```python
from build123d import *

# Parameters (mm, degrees)
SKETCH1_R           = 1.5
SKETCH1_R_2         = 1
BOSS_EXTRUDE1_DEPTH = 5
FILLET1_R           = 20
CUT_EXTRUDE1_START  = -2.5
CUT_EXTRUDE1_DEPTH  = 2.5
FILLET5_R           = 15
FILLET6_R           = 4
CHAMFER1_SIZE       = 1.5


with BuildPart() as part:
    # Sketch1 → Boss-Extrude1 (new body)
    with BuildSketch(Plane(origin=(0, 0, 0), x_dir=(1, 0, 0), z_dir=(0, 1, 0))):
        with BuildLine():
            Line((0.6, -5.969924623), (50.1, -0.994987437))
            Line((50.1, -0.994987437), (60.292075574, -4.699254638))
            ThreePointArc((60.292075574, -4.699254638), (66.917086627, -0.906785038), (62.080644677, 4.999349601))
            Line((62.080644677, 4.999349601), (0.105263158, 5.999076568))
            ThreePointArc((0.105263158, 5.999076568), (-2.95430253, 5.222269292), (-5.196152423, 3))
            Line((-5.196152423, 3), (-13.5, 3))
            ThreePointArc((-13.5, 3), (-16.5, 0), (-13.5, -3))
            Line((-13.5, -3), (-5.196152423, -3))
            ThreePointArc((-5.196152423, -3), (-2.736104409, -5.339825153), (0.6, -5.969924623))
        make_face()
        with Locations(Location((0, 0, 0), (0, 0, 270))):
            Circle(SKETCH1_R, mode=Mode.SUBTRACT)
        with Locations(Location((-13.5, 0, 0), (0, 0, 270))):
            Circle(SKETCH1_R_2, mode=Mode.SUBTRACT)
    extrude(amount=BOSS_EXTRUDE1_DEPTH)

    # Fillet1
    fillet1_edges = [part.edges().sort_by_distance(p)[0] for p in [
        (50.1, 2.5, 0.994987437),
    ]]
    fillet(fillet1_edges, radius=FILLET1_R)

    # Sketch2 → Cut-Extrude1 (cut)
    with BuildSketch(Plane(origin=(0, 5, 0), x_dir=(1, 0, 0), z_dir=(0, 1, 0)).offset(CUT_EXTRUDE1_START)):
        with BuildLine():
            Line((-13.5, 3), (-7.5, 3))
            Line((-7.5, 3), (-7.5, -3))
            Line((-7.5, -3), (-13.5, -3))
            ThreePointArc((-13.5, -3), (-16.5, 0), (-13.5, 3))
        make_face()
    extrude(amount=CUT_EXTRUDE1_DEPTH, mode=Mode.SUBTRACT)

    # Fillet5
    # the kernel refuses this fillet: 15 mm, written as the material it adds along each edge
    with BuildSketch(Plane(origin=(-5.196152423, 0, 3), x_dir=(0.7008923394400669, 0, 0.7132670807728548), z_dir=(0, 1, 0))) as fillet5_piece_1_section:
        with BuildLine():
            CenterArc((6.759639834, -14.52230372), FILLET5_R, 104.498640433, 31.002719134)
            Line((-3.939366378, -4.008918629), (0, 0))
            ThreePointArc((0, 0), (1.502142185, -0.191078512), (3.004284371, 0))
        make_face()
    fillet5_piece_1 = extrude(amount=5, mode=Mode.PRIVATE)
    fillet5_piece_1 = split(fillet5_piece_1, bisect_by=Plane(origin=(-7.5, 1.25, 3.544303671), z_dir=(1, 0, 0)), keep=Keep.TOP, mode=Mode.PRIVATE)
    fillet5_piece_1 = split(fillet5_piece_1, bisect_by=Plane(origin=(-5.459248891, 2.5, 3.544303671), z_dir=(0, -1, 0)), keep=Keep.TOP, mode=Mode.PRIVATE)
    add(fillet5_piece_1)
    with BuildSketch(Plane(origin=(-5.196152423, 0, 3), x_dir=(0.7008923394400669, 0, 0.7132670807728548), z_dir=(0, 1, 0))) as fillet5_piece_2_section:
        with BuildLine():
            CenterArc((6.759639834, -14.52230372), FILLET5_R, 104.498640433, 31.002719134)
            Line((-3.939366378, -4.008918629), (0, 0))
            ThreePointArc((0, 0), (1.502142185, -0.191078512), (3.004284371, 0))
        make_face()
    fillet5_piece_2 = extrude(amount=5, mode=Mode.PRIVATE)
    fillet5_piece_2 = split(fillet5_piece_2, bisect_by=Plane(origin=(-7.5, 1.25, 2.925994162), z_dir=(-1, 0, 0)), keep=Keep.TOP, mode=Mode.PRIVATE)
    fillet5_piece_2 = split(fillet5_piece_2, bisect_by=Plane(origin=(-8.916431377, 2.5, 2.925994162), z_dir=(0, -1, 0)), keep=Keep.TOP, mode=Mode.PRIVATE)
    add(fillet5_piece_2)
    with BuildSketch(Plane(origin=(-5.196152423, 0, 3), x_dir=(0.7008923394400669, 0, 0.7132670807728548), z_dir=(0, 1, 0))) as fillet5_piece_3_section:
        with BuildLine():
            CenterArc((6.759639834, -14.52230372), FILLET5_R, 104.498640433, 31.002719134)
            Line((-3.939366378, -4.008918629), (0, 0))
            ThreePointArc((0, 0), (1.502142185, -0.191078512), (3.004284371, 0))
        make_face()
    fillet5_piece_3 = extrude(amount=5, mode=Mode.PRIVATE)
    fillet5_piece_3 = split(fillet5_piece_3, bisect_by=Plane(origin=(-7.5, 3.75, 3.544303671), z_dir=(1, 0, 0)), keep=Keep.TOP, mode=Mode.PRIVATE)
    fillet5_piece_3 = split(fillet5_piece_3, bisect_by=Plane(origin=(-5.459248891, 2.5, 3.544303671), z_dir=(0, 1, 0)), keep=Keep.TOP, mode=Mode.PRIVATE)
    add(fillet5_piece_3)
    with BuildSketch(Plane(origin=(-5.196152423, 0, -3), x_dir=(-1, 0, 0), z_dir=(0, 1, 0))) as fillet5_piece_4_section:
        with BuildLine():
            CenterArc((5.620501404, -15), FILLET5_R, 90, 31.002719134)
            ThreePointArc((-2.105679901, -2.142857143), (-0.916549938, -1.205354037), (0, 0))
            Line((0, 0), (5.620501404, 0))
        make_face()
    fillet5_piece_4 = extrude(amount=5, mode=Mode.PRIVATE)
    fillet5_piece_4 = split(fillet5_piece_4, bisect_by=Plane(origin=(-8.916431377, 2.5, -2.925994162), z_dir=(0, -1, 0)), keep=Keep.TOP, mode=Mode.PRIVATE)
    fillet5_piece_4 = split(fillet5_piece_4, bisect_by=Plane(origin=(-7.5, 1.25, -2.925994162), z_dir=(-1, 0, 0)), keep=Keep.TOP, mode=Mode.PRIVATE)
    add(fillet5_piece_4)
    with BuildSketch(Plane(origin=(-5.196152423, 0, -3), x_dir=(-1, 0, 0), z_dir=(0, 1, 0))) as fillet5_piece_5_section:
        with BuildLine():
            CenterArc((5.620501404, -15), FILLET5_R, 90, 31.002719134)
            ThreePointArc((-2.105679901, -2.142857143), (-0.916549938, -1.205354037), (0, 0))
            Line((0, 0), (5.620501404, 0))
        make_face()
    fillet5_piece_5 = extrude(amount=5, mode=Mode.PRIVATE)
    fillet5_piece_5 = split(fillet5_piece_5, bisect_by=Plane(origin=(-5.459248891, 2.5, -3.544303671), z_dir=(0, -1, 0)), keep=Keep.TOP, mode=Mode.PRIVATE)
    fillet5_piece_5 = split(fillet5_piece_5, bisect_by=Plane(origin=(-7.5, 1.25, -3.544303671), z_dir=(1, 0, 0)), keep=Keep.TOP, mode=Mode.PRIVATE)
    add(fillet5_piece_5)
    with BuildSketch(Plane(origin=(-5.196152423, 0, -3), x_dir=(-1, 0, 0), z_dir=(0, 1, 0))) as fillet5_piece_6_section:
        with BuildLine():
            CenterArc((5.620501404, -15), FILLET5_R, 90, 31.002719134)
            ThreePointArc((-2.105679901, -2.142857143), (-0.916549938, -1.205354037), (0, 0))
            Line((0, 0), (5.620501404, 0))
        make_face()
    fillet5_piece_6 = extrude(amount=5, mode=Mode.PRIVATE)
    fillet5_piece_6 = split(fillet5_piece_6, bisect_by=Plane(origin=(-5.459248891, 2.5, -3.544303671), z_dir=(0, 1, 0)), keep=Keep.TOP, mode=Mode.PRIVATE)
    fillet5_piece_6 = split(fillet5_piece_6, bisect_by=Plane(origin=(-7.5, 3.75, -3.544303671), z_dir=(1, 0, 0)), keep=Keep.TOP, mode=Mode.PRIVATE)
    add(fillet5_piece_6)

    # Fillet6
    fillet6_edges = [part.edges().sort_by_distance(p)[0] for p in [
        (-7.5, 3.75, 3.371267745),
        (-7.5, 3.75, -3.371267745),
    ]]
    fillet(fillet6_edges, radius=FILLET6_R)

    # Chamfer1
    chamfer1_edges = [part.edges().sort_by_distance(p)[0] for p in [
        (-4.047431746, 5, -4.614275051),
        (-6.828767993, 5, -2.683225442),
        (-7.5, 5, 0),
        (-6.828767993, 5, 2.683225442),
        (-4.047431746, 5, 4.614275051),
        (-1.312106512, 5, 5.854773821),
        (23.079157013, 5, 3.710684337),
        (50.036282779, 5, 1.505294708),
        (57.341043652, 5, 3.62671444),
        (66.917086627, 5, 0.906785038),
        (31.092953917, 5, -5.499213085),
        (-1.552786741, 5, -5.795589128),
    ]]
    chamfer(chamfer1_edges, length=CHAMFER1_SIZE)


solid = part.part
```
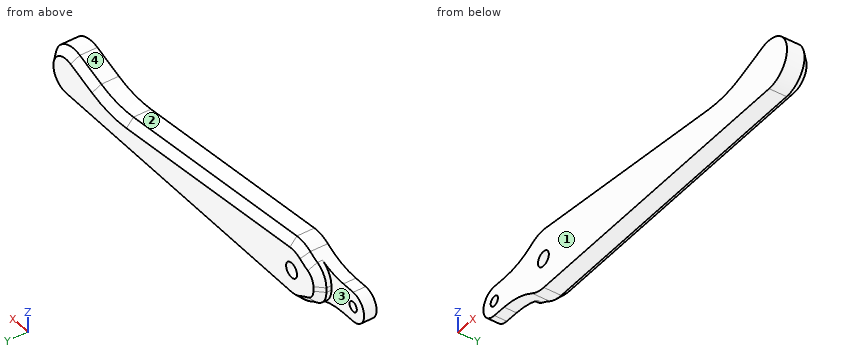
Geometry check sheet. Reference: the model listing, model coordinates, mm. Face numbers are marked on the shaded views. A direction names the side the tool comes from. Round coordinates to 2 decimals unless told otherwise and drop trailing zeros. Order: outer loops, then holes, each group sorted by start corner. A loop starts at its lowest first (then second) coordinate and runs counter-clockwise, first axis right, second up. Notation, with made-up numbers: (82.5, 5.25) -> (121.5, 5.25) arc R20 ccw to (121.5, 12.25) -> close; hole circle Ø5 at (-20, 2). An arc over 180 degrees is marked (long way). Return JSON: item names as keys, results as strings. Group by question number.
Q1. Section check B-B, the plane x = 42. Record the boundary of the cut face in (y, z).
Q2. Material ranges on probe 1 along Z at (x, y) = (-13.5, 1.6); probe 2 along X at (y, z) = (1.5, 0); probe 3 along X at (y, z) = (2.7, 0), recorded low to high. Write a range as from..to.
Q3. Release check for a two-part mould opening along X. For the marked faces 3 and 4 record: released by +X, released by -X, zero draft, split by the parting line, or undercut.
Q4. Gauge pin test, flat ends, axial feed: pin 1 (3 mm diameter, centred on x = -12, y = 1, fed in from +Z); pin 2 (3 mm diameter, centred on y = 3.5, z = -2, fed in from -X); pin 3 (6 mm diameter, centred on x = -7.5, z = -1, fed in from +Y); pin 4 (1.2 mm diameter, centred on x = -13.5, z = 0, fed in from -Y). Record the tip position at first contact, or that the pin passes through.
Q5. Tool access check on the marked faces 1 and 2. Record the directions out of +Z, -Z, +X, -X, +Y, -Y that give a thin tool (end or side, any length) a straight path to the whole face; none if there is none.
Q6. Section check C-C, the plane x = -10. Record the boundary of the cut face in (y, z).
Q7. Section check A-A, the plane y = 1.05. Record the boundary of the cut face in (x, z), plus the area to 3 significant figures.
Q8. Section check D-D, the plane x = 12.5. Record the boundary of the cut face in (y, z), plus the area to 3 significant figures.
Numbers:
{
 "1": {"outline": "(0, -5.32) -> (3.5, -5.32) -> (5, -3.82) -> (5, 0.3) -> (3.5, 1.81) -> (0, 1.81) -> close"},
 "2": {"probe 1": "-3..-1, 1..3", "probe 2": "-16.5..-14.5, -12.5..-1.5, 1.5..67", "probe 3": "-7.5..-1.5, 1.5..67"},
 "3": {"face 3": "zero draft", "face 4": "undercut"},
 "4": {"pin 1": "z = 3", "pin 2": "x = -16.37", "pin 3": "y = 5", "pin 4": "through"},
 "5": {"face 1": "+Z, -Z, +X, -X, -Y", "face 2": "+Z, +Y, -Y"},
 "6": {"outline": "(0, -3.02) -> (2.5, -3.02) -> (2.5, 3.02) -> (0, 3.02) -> close"},
 "7": {"outline": "(-13.5, -3) -> (-10.82, -3) arc R15 cw to (-3.09, -5.14) arc R6 ccw to (0.11, -6) -> (62.08, -5) arc R5 ccw (long way) to (60.29, 4.7) -> (54.39, 2.55) arc R20 cw to (45.56, 1.45) -> (0.6, 5.97) arc R6 ccw to (-3.09, 5.14) arc R15 cw to (-10.82, 3) -> (-13.5, 3) arc R3 ccw to start; hole circle Ø2 at (-13.5, 0); hole circle Ø3 at (0, 0)", "area": "708 mm^2"},
 "8": {"outline": "(0, -5.8) -> (3.5, -5.8) -> (5, -4.3) -> (5, 3.27) -> (3.5, 4.77) -> (0, 4.77) -> close", "area": "50.6 mm^2"}
}
